Can you work these out from the model? Positions are in its coordinate system, mm. Face numbers are marked on the shaded views. A direction names the side the tool comes from. Round coordinates to 2 decimals unless told otherwise and drop trailing zeros. Loops run counter-clockwise (first coordinate to the right, second up) from the corner with the lowest first, then second, coordinate; pieces in that order, holes last. Notation, with made-up numbers: (82.25, -15) - (113.25, -15) arc R34 cw to (113.25, 22) - close; hole circle Ø4 at (37.25, 32.5). An arc over 180 degrees is marked (long way). Answer as CSV lines item,"result".
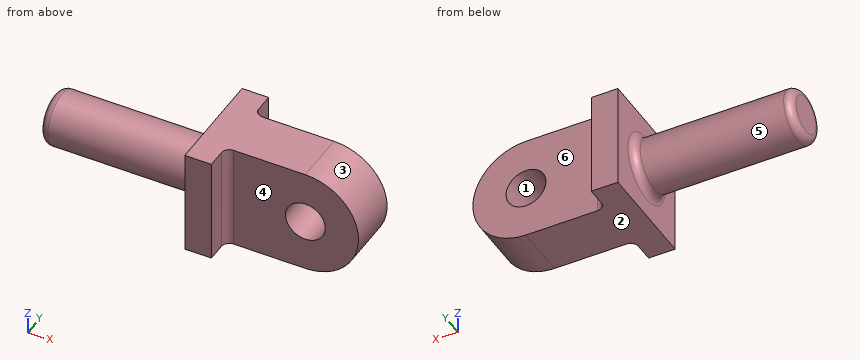
```python
from build123d import *

# Parameters (mm, degrees)
F0_W     = 50.8
F0_H     = 50.8
F1_DEPTH = 12.7
F2_R     = 12.7
F3_DEPTH = 76.2
F4_R     = 9.525
F5_DEPTH = 38.1
F6_DEPTH = 12.7
F7_R     = 3.81


with BuildPart() as f1:
    # F0 (on Right) → F1 (new body)
    with BuildSketch(Plane.YZ):
        Rectangle(F0_W, F0_H)
    extrude(amount=F1_DEPTH)

    # F2 (on face) → F3 (join)
    with BuildSketch(Plane(origin=(0, 0, 0), x_dir=(0, -1, 0), z_dir=(-1, 0, 0))):
        Circle(F2_R)
    extrude(amount=F3_DEPTH)

    # F4 (on face) → F5 (join)
    with BuildSketch(Plane.XZ.offset(25.4)):
        with BuildLine():
            Line((50.8, 25.4), (12.7, 25.4))
            Line((12.7, 25.4), (12.7, -25.4))
            Line((12.7, -25.4), (50.8, -25.4))
            ThreePointArc((50.8, -25.4), (76.2, 0), (50.8, 25.4))
        make_face()
        with Locations((50.8, 0)):
            Circle(F4_R, mode=Mode.SUBTRACT)
    extrude(amount=-F5_DEPTH)

    # F4 (on face) → F6 (cut)
    with BuildSketch(Plane.XZ.offset(25.4)):
        with BuildLine():
            Line((50.8, 25.4), (12.7, 25.4))
            Line((12.7, 25.4), (12.7, -25.4))
            Line((12.7, -25.4), (50.8, -25.4))
            ThreePointArc((50.8, -25.4), (76.2, 0), (50.8, 25.4))
        make_face()
        with Locations((50.8, 0)):
            Circle(F4_R, mode=Mode.SUBTRACT)
    extrude(amount=-F6_DEPTH, mode=Mode.SUBTRACT)

    # F7
    f7_edges = [f1.edges().sort_by_distance(p)[0] for p in [
        (-76.2, 12.7, 0),
        (0, 12.7, 0),
        (12.7, -12.7, 0),
        (12.7, 12.7, 0),
    ]]
    fillet(f7_edges, radius=F7_R)


solid = f1.part
```
Q1. Imagine slicing it at D-D (z = -18). Write out the boundary of the cut face in (x, y).
Checks:
outline,"(0, -25.4) - (12.7, -25.4) - (12.7, -16.51) arc R3.81 cw to (16.51, -12.7) - (68.72, -12.7) - (68.72, 12.7) - (16.51, 12.7) arc R3.81 cw to (12.7, 16.51) - (12.7, 25.4) - (0, 25.4) - close"
Q2. If I drill on line 1 along Z through (x, y) = (50, -3); line 2 along X through (y, z) = (-19, 8.5); line 3 along Z through (x, y) = (56.5, 6.5), over which ranges is the centre line in solid material (lowest first)? Write a range as [from, to].
Checks:
line 1,"[-25.4, -9.49], [9.49, 25.4]"
line 2,"[0, 12.7]"
line 3,"[-24.75, -7.63], [7.63, 24.75]"
Q3. Imagine slicing it at B-B (y = 0). Write out the boundary of the cut face in (x, z) (3 decimals), then the cut area to 3 significant figures.
Checks:
outline,"(-76.2, -8.89) arc R3.81 ccw to (-72.39, -12.7) - (-3.81, -12.7) arc R3.81 cw to (0, -16.51) - (0, -25.4) - (50.8, -25.4) arc R25.4 ccw to (50.8, 25.4) - (0, 25.4) - (0, 16.51) arc R3.81 cw to (-3.81, 12.7) - (-72.39, 12.7) arc R3.81 ccw to (-76.2, 8.89) - close; hole circle Ø19.05 at (50.8, 0)"
area,"5,240 mm²"
Q4. Imagine slicing it at A-A (z = 0). Write out the boundary of the cut face in (x, y) (3 decimals), then the cut area to 3 significant figures.
Checks:
outline,"(-76.2, -8.89) arc R3.81 ccw to (-72.39, -12.7) - (-3.81, -12.7) arc R3.81 cw to (0, -16.51) - (0, -25.4) - (12.7, -25.4) - (12.7, -16.51) arc R3.81 cw to (16.51, -12.7) - (41.275, -12.7) - (41.275, 12.7) - (16.51, 12.7) arc R3.81 cw to (12.7, 16.51) - (12.7, 25.4) - (0, 25.4) - (0, 16.51) arc R3.81 cw to (-3.81, 12.7) - (-72.39, 12.7) arc R3.81 ccw to (-76.2, 8.89) - close; (60.325, -12.7) - (76.2, -12.7) - (76.2, 12.7) - (60.325, 12.7) - close"
area,"3,720 mm²"
Q5. Imagine slicing it at C-C (x = -31). Write out the boundary of the cut face in (y, z).
Checks:
outline,"circle Ø25.4 at (0, 0)"
Q6. I'm going to push flat-ended pins straight in: pin 1 Ø15 at (x, z) = (32, -0.5) entering from +Y; pin 2 Ø7 at (y, z) = (21, 4) entering from +X; pin 3 Ø1 at (y, z) = (-17.5, -17.5) entering from -X. Where does each tip first touch, or does it pass through?
Checks:
pin 1,"y = 12.7"
pin 2,"x = 12.7"
pin 3,"x = 0"
Q7. We'd pull the mould along Z, two halves only. Please class the marked faces 1, 2 and 3: pulls with the +Z half, pulls with the -Z half, needs draft (parallel to the pull), parting line crosses it, or undercut.
Checks:
face 1,"undercut"
face 2,"pulls with the -Z half"
face 3,"parting line crosses it"
Q8. On a 3-axis mill with a long thin cutter (end or side, diameter ignored), from which of +Z, -Z, +X, -X, +Y, -Y can I reach the whole of each face in a straight line? I mean the marked faces 4, 5 and 6. Say none if no direction works.
Checks:
face 4,"+Z, -Z, +X, -Y"
face 5,"-X"
face 6,"+Z, -Z, +X, +Y"
